Autodesk Inventor part; units mm, degrees
ref_plane "YZ Plane" through (0, 0, 0) normal (1, 0, 0) x (0, 1, 0)
ref_plane "XZ Plane" through (0, 0, 0) normal (0, 1, 0) x (-1, 0, 0)
ref_plane "XY Plane" through (0, 0, 0) normal (0, 0, 1) x (1, 0, 0)
sketch "Sketch1" plane through (0, 0, 0) normal (0, 1, 0) x (-1, 0, 0)
  line L0 (0, 0) -> (-16, 0)
  line L1 (-16, 0) -> (-16, -16)
  line L2 (-16, -16) -> (0, -16)
  line L3 (0, -16) -> (0, 0)
  dimension "d0" = 16
extrude "Extrusion1" add sketch "Sketch1" along normal blind 12
sketch "Sketch2" plane through (16, 0, -16) normal (0, 0, -1) x (-1, 0, 0)
  line L0 (16, 0) -> (16, 12)
  line L1 (0, 12) -> (16, 12)
  circle A0 centre (11, 7.3) radius 3
  dimension "d3" = 6
  dimension "d4" = 5
  dimension "d5" = 4.7
extrude "Extrusion2" cut sketch "Sketch2" against normal through all
sketch "Sketch3" plane through (0, 0, 0) normal (0, 0, 1) x (1, 0, 0)
  line L0 (0, 0) -> (16, 0)
  line L1 (16, 0) -> (16, 12)
  point P0 (13.9, 2.1)
  dimension "d8" = 2.1
  dimension "d9" = 2.1
hole "Hole1" at (13.9, 2.1, 0) direction (0, 0, -1) diameter 2 depth 5 tip angle 118 countersink diameter 2.5 countersink angle 90
sketch "Sketch4" plane through (0, 12, 0) normal (0, 1, 0) x (1, 0, 0)
  line L0 (16, 0) -> (16, 16)
  line L1 (0, 16) -> (0, 0)
  circle A0 centre (11.5, 8) radius 2.5
  point P0 (0, 8)
  dimension "d17" = 5
  dimension "d18" = 4.5
extrude "Extrusion3" cut sketch "Sketch4" against normal through all
sketch "Sketch5" plane through (0, 0, -16) normal (-1, 0, 0) x (0, 0, 1)
  line L0 (0, 12) -> (16, 12)
  line L1 (0, 4.3) -> (0, 10.3)
  line L2 (16, 10.3) -> (16, 4.3)
  line L3 (0, 4.3) -> (0, 10.3)
  line L4 (0, 7.3) -> (16, 7.3) construction
  circle A0 centre (8, 7.3) radius 1
  dimension "d21" = 4.7
  dimension "d22" = 2
extrude "Extrusion4" cut sketch "Sketch5" against normal up to surface
thread "Thread1"
chamfer "Chamfer1" distance 0.2 angle 45 1 edges at (0, 7.3, -9)
chamfer "Chamfer2" distance 0.2 angle 45 2 edges at (8, 7.3, 0) (8, 7.3, -16)
properties part number "heatblock" material "Aluminum 6061"
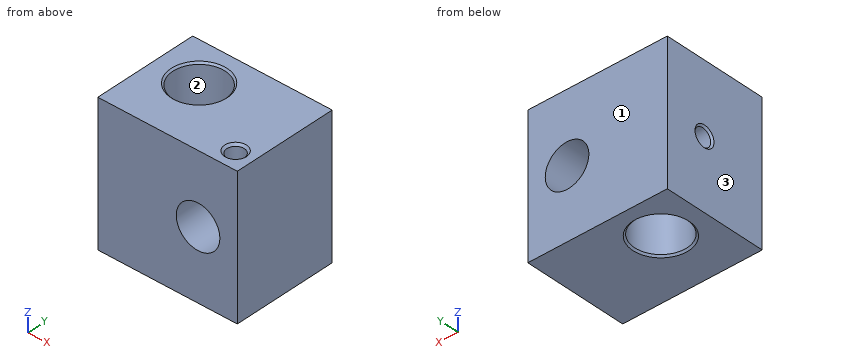
Geometry check sheet. Reference: the model listing, model coordinates, mm. Face numbers are marked on the shaded views. Coordinates: 2 decimals unless noted, no trailing zeros. Order: outer loops, then holes, each group sorted by start corner. A loop starts at its lowest first (then second) coordinate and runs counter-clockwise, first axis right, second up. Notation, with made-up numbers: M 13.5,56.25 L 28.5,56.25 A35 cw 28.5,92.25 Z; hole C 44.25,-18.75 d9. An arc over 180 degrees is marked long. One line per question, with ' | ' between items. Start each with the question number.
Item 1: Gauge pin test, flat end, axial feed: pin 1 (5 mm diameter, centred on x = 12, z = -8.5, fed in from +Y). Record the tip position at first contact, or that the pin passes through.
Item 2: Draft check along Y on the marked faces 1, 2 and 3. Enter one of: pulls with the +Y half, pulls with the -Y half, needs draft (parallel to the pull), parting line crosses it, or undercut.
Item 3: Cross-section at B-B on y = 6.75. State how many separate pieces and enclosed holes the cut face has, then the cut area to 3 significant figures.
Item 4: Material ranges on L1, parallel to Y at x = 13.9, z = -1.45; L2, parallel to Z at x = 1.5, y = 7.3; L3, parallel to Y at x = 5, z = -4.75, recorded low to high. Write a range as [from, to].
Item 5: Cross-section at A-A on x = 5. Enter the section's corners in (y, z), then the cut area to 3 significant figures.
Item 6: Cross-section at D-D on z = -2.75. Enter the section's corners in (x, y), then the cut area to 3 significant figures.
Item 7: Cross-section at C-C on x = 10. Enter the section's corners in (y, z), then the cut area to 3 significant figures.
Findings:
1) pin 1: stops at y = 12
2) face 1: pulls with the +Y half | face 2: undercut | face 3: needs draft
3) separate pieces: 3 | enclosed holes: 1 | area: 138 mm²
4) L1: y = [0, 1.1], [3.1, 12] | L2: z = [-16, -9], [-7, 0] | L3: y = [0, 4.3], [10.3, 12]
5) outline: M 0,-16 L 4.1,-16 L 4.3,-15.8 L 4.3,-0.2 L 4.1,0 L 0,0 Z; M 10.3,-15.8 L 10.5,-16 L 12,-16 L 12,0 L 10.5,0 L 10.3,-0.2 Z | area: 95.9 mm²
6) outline: M 0,0 L 16,0 L 16,12 L 0,12 Z; hole C 5,7.3 d6; hole C 13.9,2.1 d2 | area: 161 mm²
7) outline: M 0,-16 L 12,-16 L 12,-10 L 0,-10 Z; M 0,-6 L 12,-6 L 12,0 L 0,0 Z | area: 144 mm²
